Verification items for the finished model (mm, model axes). A direction names the side the tool comes from. Give positions to 0.01 mm unless a question says otherwise; leave off trailing zeros. Order: outer loops, then holes, each group sorted by start corner. A loop starts at its lowest first (then second) coordinate and runs counter-clockwise, first axis right, second up.
from build123d import *

# Parameters (mm, degrees)
F1_DEPTH = 40


with BuildPart() as f1:
    # F0 (on Front) → F1 (new body)
    with BuildSketch(Plane.XZ):
        with BuildLine():
            Line((0, 0), (-50, 0))
            Line((-50, 0), (-50, -3))
            ThreePointArc((-50, -3), (-49.707107, -3.707107), (-49, -4))
            Line((-49, -4), (-46, -4))
            Line((-46, -4), (-45, -3))
            Line((-45, -3), (-44, -4))
            Line((-44, -4), (-40, -4))
            ThreePointArc((-40, -4), (-32.928932, -6.928932), (-30, -14))
            Line((-30, -14), (-30, -40))
            ThreePointArc((-30, -40), (-27.071068, -47.071068), (-20, -50))
            Line((-20, -50), (-11, -50))
            ThreePointArc((-11, -50), (-10.292893, -49.707107), (-10, -49))
            Line((-10, -49), (-10, -40.57735))
            ThreePointArc((-10, -40.57735), (-10.5, -39.711325), (-11.5, -39.711325))
            Line((-11.5, -39.711325), (-18, -43.464102))
            ThreePointArc((-18, -43.464102), (-23.464102, -42), (-22, -36.535898))
            Line((-22, -36.535898), (-10.5, -29.89637))
            ThreePointArc((-10.5, -29.89637), (-10.133975, -29.530345), (-10, -29.030345))
            Line((-10, -29.030345), (-10, -5))
            ThreePointArc((-10, -5), (-9.707107, -4.292893), (-9, -4))
            Line((-9, -4), (-6, -4))
            Line((-6, -4), (-5, -3))
            Line((-5, -3), (-4, -4))
            Line((-4, -4), (-1, -4))
            ThreePointArc((-1, -4), (-0.292893, -3.707107), (0, -3))
            Line((0, -3), (0, 0))
        make_face()
    extrude(amount=-F1_DEPTH)


solid = f1.part
(1) Section check B-B, the plane y = 27. Enter the section's corners in (x, z), then the cut area to 3 significant figures.
Solved:
outline: (-50, -3) arc R1 ccw to (-49, -4) - (-46, -4) - (-45, -3) - (-44, -4) - (-40, -4) arc R10 cw to (-30, -14) - (-30, -40) arc R10 ccw to (-20, -50) - (-11, -50) arc R1 ccw to (-10, -49) - (-10, -40.58) arc R1 ccw to (-11.5, -39.71) - (-18, -43.46) arc R4 cw to (-22, -36.54) - (-10.5, -29.9) arc R1 ccw to (-10, -29.03) - (-10, -5) arc R1 cw to (-9, -4) - (-6, -4) - (-5, -3) - (-4, -4) - (-1, -4) arc R1 ccw to (0, -3) - (0, 0) - (-50, 0) - close
area: 999 mm2
(2) Section check A-A, the plane z = -42. Enter the section's corners in (x, y).
Solved:
outline: (-29.8, 0) - (-23.46, 0) - (-23.46, 40) - (-29.8, 40) - close; (-15.46, 0) - (-10, 0) - (-10, 40) - (-15.46, 40) - close
(3) Go/stop test with flat-tipped pins: pin 1 (4 mm diameter, centred on y = 23, z = -44, fed in from +X); pin 2 (0.9 mm diameter, centred on x = -47.5, y = 27.5, fed in from -Z); pin 3 (5 mm diameter, centred on y = 19.5, z = -8.5, fed in from -X); pin 4 (1.5 mm diameter, centred on x = -10.5, y = 9.5, fed in from +Z). Record where each tip stops, or that it passes through.
Solved:
pin 1: stops at x = -10
pin 2: stops at z = -4
pin 3: stops at x = -34
pin 4: stops at z = 0
(4) Section check C-C, the plane z = -27.5. Enter the section's corners in (x, y).
Solved:
outline: (-30, 0) - (-10, 0) - (-10, 40) - (-30, 40) - close
(5) Scan lines: line 1 (Z direction, x = -3.5, y = 16); line 2 (X direction, y = 36, z = -14.5); line 3 (Z direction, x = -18.5, y = 38.5). Record each from-to range of solid material in increasing order.
Solved:
line 1: z = -4 to 0
line 2: x = -30 to -10
line 3: z = -50 to -43.71, -34.52 to 0
(6) Section check D-D, the plane x = -39. Enter the section's corners in (y, z), then the cut area to 3 significant figures.
Solved:
outline: (0, -4.05) - (40, -4.05) - (40, 0) - (0, 0) - close
area: 162 mm2
(7) Release check for a two-part mould opening along Z. For faces 1 (the flat face through (-8, 20, -4)), 2 (the cylindrical face through (-10.487, 19.72, -39.719)), 3 (the flat face through (-25, 20, 0)) record: pulls with the +Z half, pulls with the -Z half, needs draft (parallel to the pull), parting line crosses it, or undercut.
Solved:
face 1: pulls with the -Z half
face 2: undercut
face 3: pulls with the +Z half
(8) Set-up check for faces 4 (the flat face through (-10, 20, -45)), 5 (the flat face through (-14.7, 19.72, -41.56)), 6 (the flat face through (-48, 20, -4)), 7 (the flat face through (-16.33, 19.72, -33.263)): record each of +Z, -Z, +X, -X, +Y, -Y from which the full face is reachable in a straight line by a thin tool's end or side.
Solved:
face 4: -Z, +X, +Y, -Y
face 5: +Y, -Y
face 6: -Z, -X, +Y, -Y
face 7: +X, +Y, -Y
